Verification items for this drawing (mm, ordinates from the low corner). A direction names the side the tool comes from. Coordinates: 2 decimals unless noted, no trailing zeros. Order: outer loops, then holes, each group sorted by start corner. A loop starts at its lowest first (then second) coordinate and runs counter-clockwise, first axis right, second up. Notation, with made-up numbers: M 69,5.5 L 106,5.5 A18 cw 106,37.5 Z; hole C -12.75,-10.75 d5. An arc over 180 degrees is marked long. Answer as a JSON object with one key per item and string values. Group by question number.
(1) Material ranges on line 1 (Y direction, x = 15, z = 24); line 2 (X direction, y = 12, z = 21.75); line 3 (X direction, y = 19.5, z = 6.5), recorded low to high.
(2) Cross-section at B-B (y = 6.5). Enter the section's corners in (x, z), plus the area to 3 significant figures.
(3) Access from +Z, -Z, +X, -X, +Y, -Y to the whole of each face (thin tool, end or side, straight path). Record for the marked faces 1 and 2.
(4) Cross-section at A-A (x = 125). Enter the section's corners in (y, z), plus the area to 3 significant figures.
(5) Gauge pin test, flat ends, axial feed: pin 1 Ø2 at (y, z) = (26, 12) entering from -X; pin 2 Ø4 at (y, z) = (9.5, 16) entering from +X; pin 3 Ø8 at (y, z) = (8.5, 23.5) entering from -X. Record the tip position at first contact, or that the pin passes through.
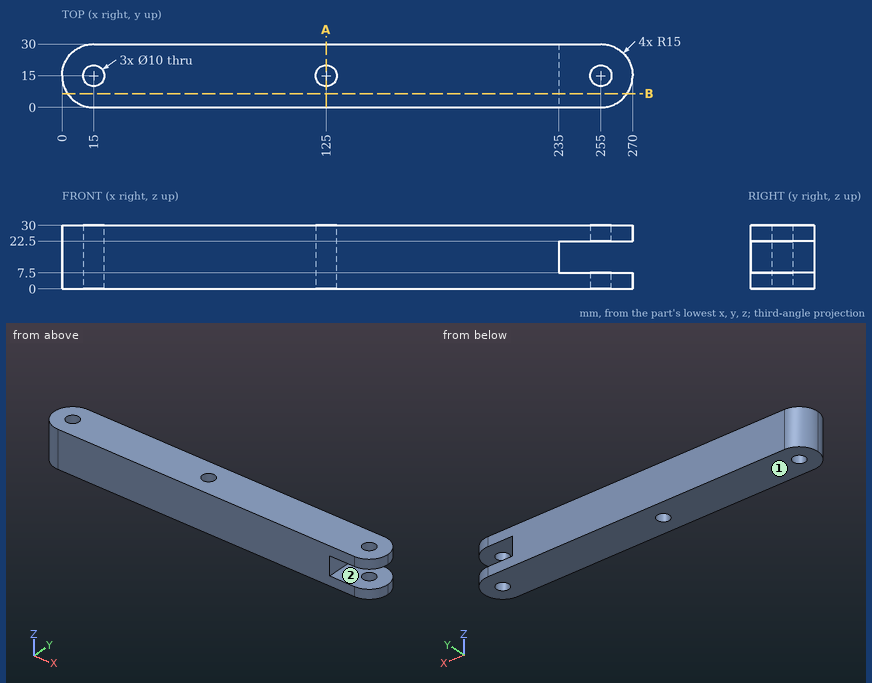
Taken from the geometry:
{
 "1": {"line 1": "y = 0 to 10, 20 to 30", "line 2": "x = 0.3 to 11, 19 to 121, 129 to 235", "line 3": "x = 0.69 to 12.82, 17.18 to 122.82, 127.18 to 252.82, 257.18 to 269.31"},
 "2": {"outline": "M 2.64,0 L 267.36,0 L 267.36,7.5 L 235,7.5 L 235,22.5 L 267.36,22.5 L 267.36,30 L 2.64,30 Z", "area": "7,460 mm²"},
 "3": {"face 1": "-Z, +X, -X, +Y, -Y", "face 2": "+X, +Y, -Y"},
 "4": {"outline": "M 0,0 L 10,0 L 10,30 L 0,30 Z; M 20,0 L 30,0 L 30,30 L 20,30 Z", "area": "600 mm²"},
 "5": {"pin 1": "stops at x = 3.82", "pin 2": "stops at x = 235", "pin 3": "stops at x = 0.21"}
}
